Print and shaded views of the part. All mm, measured from the part's lowest x, y and z. Give positions to 0.01 mm unless a question says otherwise; leave off trailing zeros. Write each loop counter-clockwise with the first axis right and the second up, starting at its lowest first coordinate (ties: lowest second). Pieces come first, ordered by that corner, then holes. Notation, with made-up numbers: M 2,18.25 L 14,18.25 A31 cw 14,46.25 Z; hole C -30,-8 d7. An arc over 180 degrees is marked long. One line per question, with ' | ' between items. Start each with the question number.
1. Cut at B-B, the plane x = 12. Write the cut outline in (y, z).
2. Cut at A-A, the plane z = 10. Write the cut outline in (x, y).
3. Cut at C-C, the plane y = 26. Write the cut outline in (x, z), then the cut area to 3 significant figures.
4. Flat gauge pin, fed straight in: pin 1 (1.5 mm diameter, centred on x = 86, z = 10.5, fed in from +Y). Where does the tip first touch, or does it go through?
5. Wall check: L1, parallel to X at y = 11, z = 15.5; L2, parallel to Y at x = 48, z = 16; L3, parallel to Z at x = 12, y = 30. Give the ranges that are in metal, low to high.
6. Cut at D-D, the plane y = 17. Write the cut outline in (x, z), then the cut area to 3 significant figures.
7. Pull direction X, two halves, no side cores. Call the marked faces 1, 2 and 3: released by +X, released by -X, zero draft, split by the parting line, or undercut.
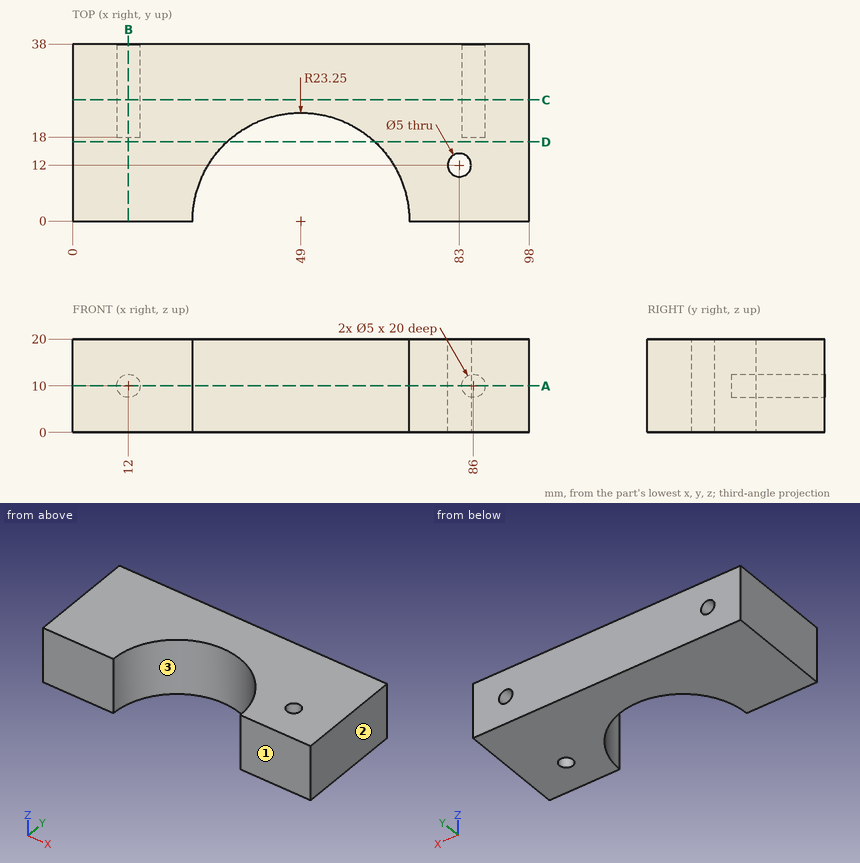
Here are the results:
1) outline: M 0,0 L 38,0 L 38,7.5 L 18,7.5 L 18,12.5 L 38,12.5 L 38,20 L 0,20 Z
2) outline: M 0,0 L 25.75,0 A23.25 cw 72.25,0 L 98,0 L 98,38 L 88.5,38 L 88.5,18 L 83.5,18 L 83.5,38 L 14.5,38 L 14.5,18 L 9.5,18 L 9.5,38 L 0,38 Z; hole C 83,12 d5
3) outline: M 0,0 L 98,0 L 98,20 L 0,20 Z; hole C 12,10 d5; hole C 86,10 d5 | area: 1,920 mm^2
4) pin 1: y = 18
5) L1: 0 to 28.52, 69.48 to 80.71, 85.29 to 98 | L2: 23.23 to 38 | L3: 0 to 7.5, 12.5 to 20
6) outline: M 0,0 L 33.14,0 L 33.14,20 L 0,20 Z; M 64.86,0 L 98,0 L 98,20 L 64.86,20 Z | area: 1,330 mm^2
7) face 1: zero draft | face 2: released by +X | face 3: undercut
